from build123d import *

# Parameters (mm, degrees)
BOSS_EXTRU_1_DEPTH      = 3
ESQUISSE2_R             = 2.6
ENL_V_MAT_EXTRU_1_DEPTH = 20


with BuildPart() as part:
    # Esquisse1 → Boss.-Extru.1 (new body)
    with BuildSketch(Plane.XY):
        Polygon((0, 450.3), (-8, 450.3), (-8, 495.3), (-59.18, 495.3), (-100, 325.5), (-100, 92.65), (-70, 0), (0, 0), align=None)
    extrude(amount=BOSS_EXTRU_1_DEPTH)

    # Esquisse2 → Enlèv. mat.-Extru.1 (cut)
    with BuildSketch(Plane(origin=(0, 0, 0), x_dir=(-1, 0, 0), z_dir=(0, 0, -1))):
        with Locations((61.335187385, 15.440747023)):
            Circle(ESQUISSE2_R)
        with Locations((85.503041698, 86.832938888)):
            Circle(ESQUISSE2_R)
        with Locations((91.66409495, 105.860325015)):
            Circle(ESQUISSE2_R)
        with Locations((88, 315.5)):
            Circle(ESQUISSE2_R)
        with Locations((88, 335.5)):
            Circle(ESQUISSE2_R)
        with Locations((51.165806832, 479.3)):
            Circle(ESQUISSE2_R)
    extrude(amount=-ENL_V_MAT_EXTRU_1_DEPTH, mode=Mode.SUBTRACT)


solid = part.part
Input: part model. Units: mm. Frame: model coordinates. Coordinates: 2 decimals unless noted, no trailing zeros. Order: outer loops, then holes, each group sorted by start corner. A loop starts at its lowest first (then second) coordinate and runs counter-clockwise, first axis right, second up.
1. Cut plane A-A, the plane z = 1.6. Return loops of the section in (x, y).
Checked values:
outline: (-100, 92.65) - (-70, 0) - (0, 0) - (0, 450.3) - (-8, 450.3) - (-8, 495.3) - (-59.18, 495.3) - (-100, 325.5) - close; hole circle Ø5.2 at (-91.66, 105.86); hole circle Ø5.2 at (-88, 315.5); hole circle Ø5.2 at (-88, 335.5); hole circle Ø5.2 at (-85.5, 86.83); hole circle Ø5.2 at (-61.34, 15.44); hole circle Ø5.2 at (-51.17, 479.3)
2. Cut plane B-B, the plane y = 425. Return loops of the section in (x, z), plus the area to 3 significant figures.
Checked values:
outline: (-76.08, 0) - (0, 0) - (0, 3) - (-76.08, 3) - close
area: 228 mm2
3. Ray query, line 1 along X through (y, z) = (107, 0.35); line 2 along Y through (x, z) = (-5.5, 1.4); line 3 along X through (y, z) = (381, 2). Return the intervals inside material, ascending.
Checked values:
line 1: x = -100 to -94, -89.33 to 0
line 2: y = 0 to 450.3
line 3: x = -86.66 to 0
